The listing builds one solid part. Answer for the finished solid, in the listing's coordinates (mm). A direction names the side the tool comes from. Give positions to 0.01 mm unless a question says otherwise; leave off trailing zeros. Write each loop counter-clockwise with the first axis right and the second up, starting at its lowest first coordinate (ties: lowest second). Pieces come first, ordered by that corner, then holes. Notation, with made-up numbers: (42.5, 76) - (59.5, 76) arc R25 ccw to (59.5, 95) - close; hole circle Ø2 at (-34.5, -36). An arc over 180 degrees is marked (long way). One line per question, with ' | ' between items. Start each with the question number.
1. A cutting plane is placed at D-D (x = 32.5). Determine the outline of the cut face in (y, z).
2. For faces 4 (the face through (40, 11.1, 27.9)), 5 (the face through (92.56, 9.88, 28.64)), 6 (the face through (20, 2.361, 28)), determine the directions among +Z, -Z, +X, -X, +Y, -Y from which every point of the face is accessible in a straight line to the end or side of a thin tool.
3. A cutting plane is placed at A-A (y = 12.5). Determine the outline of the cut face in (x, z).
4. A cutting plane is placed at B-B (x = 87.5). Determine the outline of the cut face in (y, z).
5. Find the intervals of material crossed by L1, parallel to Y at x = 44.5, z = 27; L2, parallel to X at y = 9.5, z = 19.5; L3, parallel to X at y = 11.5, z = 20, in increasing order. Write a range as from..to.
6. The mould has two halves that part along Y. Classify faces 1 (the face through (19.54, 7.27, 26.17)), 2 (the face through (94.406, 12.882, 25.773)), 3 (the face through (86, 8.361, 28)): +Y half, -Y half, draft (parallel to the pull), parting line (faces both ways), or undercut.
7. Given P1, Ø4, axis at x = 83.5, z = 30.5, coming from the -Y side; P2, Ø6, axis at y = 5.5, z = 29, coming from the +X side; P3, Ø2, axis at y = 7.78, z = 27.79, coming from the -X side, each flat-ended and moving along its own axis, determine where each tip first touches the part or whether it passes through.
8. A cutting plane is placed at C-C (z = 23.25). Determine the outline of the cut face in (x, y), then the cut area to 3 significant figures.
```python
from build123d import *

# Parameters (mm, degrees)
SKETCH_1_W      = 20
SKETCH_1_H      = 17
EXTRUDE_1_DEPTH = 40
SKETCH_2_W      = 20
SKETCH_2_H      = 5
EXTRUDE_2_DEPTH = 60
SKETCH_3_R      = 9
EXTRUDE_3_DEPTH = 3
SKETCH_4_R      = 7
EXTRUDE_4_DEPTH = 3


with BuildPart() as part:
    # Эскиз1 → Бобышка-Вытянуть1 (new body)
    with BuildSketch(Plane(origin=(0, 0, 0), x_dir=(0, 0, -1), z_dir=(1, 0, 0))):
        with Locations((-27.72412662, 10.860988518)):
            Rectangle(SKETCH_1_W, SKETCH_1_H)
    extrude(amount=EXTRUDE_1_DEPTH)

    # Эскиз2 → Бобышка-Вытянуть2 (add)
    with BuildSketch(Plane(origin=(40, 0, 0), x_dir=(0, 0, -1), z_dir=(1, 0, 0))):
        with Locations((-27.72412662, 16.860988518)):
            Rectangle(SKETCH_2_W, SKETCH_2_H)
    extrude(amount=EXTRUDE_2_DEPTH)

    # Эскиз3 → Бобышка-Вытянуть3 (add)
    with BuildSketch(Plane.XZ.offset(-14.360988518)):
        with Locations(Location((85.620234383, 27.72412662, 0), (0, 0, 90))):
            Circle(SKETCH_3_R)
    extrude(amount=EXTRUDE_3_DEPTH)

    # Эскиз4 → Бобышка-Вытянуть4 (add)
    with BuildSketch(Plane.XZ.offset(-11.360988518)):
        with Locations(Location((85.620234383, 27.72412662, 0), (0, 0, 270))):
            Circle(SKETCH_4_R)
    extrude(amount=EXTRUDE_4_DEPTH)

    # Эскиз15 → Зенковка для винта с полупотайной головкой M32 (revolve, cut)
    with BuildSketch(Plane(origin=(40, 7.784111953, 27.791024889), x_dir=(0, 0, -1), z_dir=(0, 1, 0))):
        Polygon((0, 0), (0, 40), (1.7, 40), (1.7, 1.45), (3.15, 0), align=None)
    revolve(axis=Axis((46.35, 7.784111953, 27.791024889), (-1, 0, 0)), mode=Mode.SUBTRACT)


solid = part.part
```
Determined:
1) outline: (2.36, 17.72) - (19.36, 17.72) - (19.36, 37.72) - (2.36, 37.72) - close; hole circle Ø3.4 at (7.78, 27.79)
2) face 4: +Z, -Z, -Y | face 5: -Y | face 6: +Z, -Z, +X, -X, -Y
3) outline: (0, 17.72) - (40, 17.72) - (40, 37.72) - (0, 37.72) - close; circle Ø18 at (85.62, 27.72)
4) outline: (8.36, 20.98) - (11.36, 20.98) - (11.36, 18.92) - (14.36, 18.92) - (14.36, 17.72) - (19.36, 17.72) - (19.36, 37.72) - (14.36, 37.72) - (14.36, 36.53) - (11.36, 36.53) - (11.36, 34.47) - (8.36, 34.47) - close
5) L1: 14.36..19.36 | L2: 0..40 | L3: 0..40, 81..90.24
6) face 1: undercut | face 2: draft | face 3: -Y half
7) P1: y = 8.36 | P2: x = 92.61 | P3: x = 78.62
8) outline: (0, 2.36) - (40, 2.36) - (40, 14.36) - (77.81, 14.36) - (77.81, 11.36) - (80.24, 11.36) - (80.24, 8.36) - (91, 8.36) - (91, 11.36) - (93.43, 11.36) - (93.43, 14.36) - (100, 14.36) - (100, 19.36) - (0, 19.36) - close | area: 1,060 mm2
